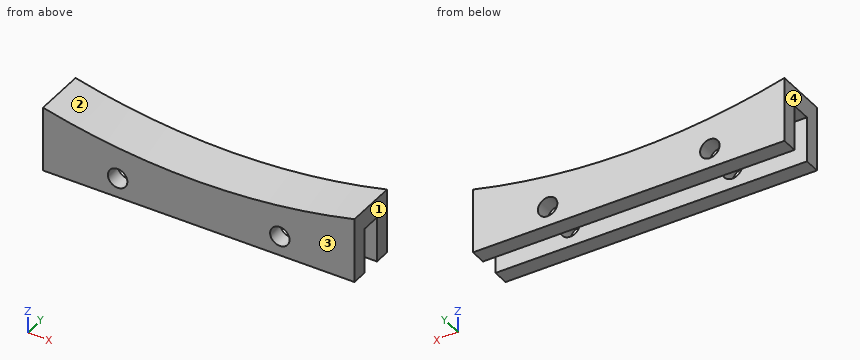
```python
from build123d import *

# Parameters (mm, degrees)
BOSS_EXTRUDE1_DEPTH = 4
SKETCH10_R          = 1.5
SKETCH10_W          = 40
SKETCH10_H          = 6.922711204
CUT_EXTRUDE2_DEPTH  = 31.436460939
SKETCH11_W          = 48
SKETCH11_H          = 1.077288796
BOSS_EXTRUDE2_DEPTH = 8
SKETCH12_W          = 7
SKETCH12_H          = 3.075
CUT_EXTRUDE3_DEPTH  = 52.052699777


with BuildPart() as part:
    # Sketch1 → Boss-Extrude1 (new, symmetric)
    with BuildSketch(Plane(origin=(0, 0, 0), x_dir=(1, 0, 0), z_dir=(0, 1, 0))):
        with BuildLine():
            Line((-20, 0), (0, 0))
            Line((0, 0), (20, 0))
            Line((20, 0), (20, -8))
            Line((20, -8), (24, -8))
            Line((24, -8), (24, -16.922711204))
            ThreePointArc((24, -16.922711204), (0, -14), (-24, -16.922711204))
            Line((-24, -16.922711204), (-24, -8))
            Line((-24, -8), (-20, -8))
            Line((-20, -8), (-20, 0))
        make_face()
    extrude(amount=BOSS_EXTRUDE1_DEPTH, both=True)

    # Sketch10 → Cut-Extrude2 (cut, through all)
    with BuildSketch(Plane(origin=(0, 4, 0), x_dir=(1, 0, 0), z_dir=(0, 1, 0))):
        with Locations(Location((-12.5, -9.922711204, 0), (0, 0, 270))):
            Circle(SKETCH10_R)
        with Locations(Location((12.5, -9.922711204, 0), (0, 0, 270))):
            Circle(SKETCH10_R)
        with Locations((0, -3.461355602)):
            Rectangle(SKETCH10_W, SKETCH10_H)
    extrude(amount=-CUT_EXTRUDE2_DEPTH, mode=Mode.SUBTRACT)

    # Sketch11 → Boss-Extrude2 (add)
    with BuildSketch(Plane(origin=(0, 4, 0), x_dir=(1, 0, 0), z_dir=(0, 1, 0))):
        with Locations((0, -7.461355602)):
            Rectangle(SKETCH11_W, SKETCH11_H)
    extrude(amount=-BOSS_EXTRUDE2_DEPTH)

    # Sketch12 → Cut-Extrude3 (cut, through all)
    with BuildSketch(Plane.ZY.offset(24)):
        with Locations((10.422711204, 0)):
            Rectangle(SKETCH12_W, SKETCH12_H)
    extrude(amount=-CUT_EXTRUDE3_DEPTH, mode=Mode.SUBTRACT)


solid = part.part
```
Design review of the part built by this model. Coordinates are the model's own, in mm. Face numbers are marked on the shaded views. Give positions to 0.01 mm unless a question says otherwise; leave off trailing zeros. Write each loop counter-clockwise with the first axis right and the second up, starting at its lowest first coordinate (ties: lowest second). Pieces come first, ordered by that corner, then holes. Notation, with made-up numbers: (84, 74.5) -> (97, 74.5) arc R6 cw to (97, 85.5) -> close; hole circle Ø7 at (-3, -17.75). An arc over 180 degrees is marked (long way). Answer in a Markdown table with one row per item.
(1) Consider section C-C (x = -12.5). State the section outline as (y, z) points.
Results:
| item | result |
|---|---|
| outline | (-4, 6.92) -> (-1.54, 6.92) -> (-1.54, 8.42) -> (-4, 8.42) -> close; (-4, 11.42) -> (-1.54, 11.42) -> (-1.54, 13.92) -> (1.54, 13.92) -> (1.54, 11.42) -> (4, 11.42) -> (4, 14.78) -> (-4, 14.78) -> close; (1.54, 6.92) -> (4, 6.92) -> (4, 8.42) -> (1.54, 8.42) -> close |
(2) Clearance check with flat-ended pins moving along their axes: pin 1 (5 mm diameter, centred on x = 12.5, z = 9.92, fed in from +Y); pin 2 (1.8 mm diameter, centred on x = 12.5, z = 9.92, fed in from -Y); pin 3 (4 mm diameter, centred on x = 15, y = -2.5, fed in from +Z); pin 4 (3 mm diameter, centred on x = 10.5, y = -3, fed in from +Z). State where each tip first meets the part, or that it passes through.
Results:
| item | result |
|---|---|
| pin 1 | y = 4 |
| pin 2 | through |
| pin 3 | z = 15.46 |
| pin 4 | z = 14.72 |
(3) Consider section D-D (z = 9). State the section outline as (x, y) points, then the cut area to 3 significant figures.
Results:
| item | result |
|---|---|
| outline | (-24, -4) -> (-13.68, -4) -> (-13.68, -1.54) -> (-24, -1.54) -> close; (-24, 1.54) -> (-13.68, 1.54) -> (-13.68, 4) -> (-24, 4) -> close; (-11.32, -4) -> (11.32, -4) -> (11.32, -1.54) -> (-11.32, -1.54) -> close; (-11.32, 1.54) -> (11.32, 1.54) -> (11.32, 4) -> (-11.32, 4) -> close; (13.68, -4) -> (24, -4) -> (24, -1.54) -> (13.68, -1.54) -> close; (13.68, 1.54) -> (24, 1.54) -> (24, 4) -> (13.68, 4) -> close |
| area | 213 mm2 |
(4) To check wall thickness, follow probe 1 along Y at (x, z) = (-2.5, 13.5); probe 2 along X at (y, z) = (2.5, 10.5); probe 3 along X at (y, z) = (3, 8.75). State the ranges of each line that lie inside material, in increasing order.
Results:
| item | result |
|---|---|
| probe 1 | -4 to -1.54, 1.54 to 4 |
| probe 2 | -24 to -13.88, -11.12 to 11.12, 13.88 to 24 |
| probe 3 | -24 to -13.44, -11.56 to 11.56, 13.44 to 24 |
(5) Consider section B-B (y = -2). State the section outline as (x, z) points.
Results:
| item | result |
|---|---|
| outline | (-24, 6.92) -> (24, 6.92) -> (24, 16.92) arc R100 cw to (-24, 16.92) -> close; hole circle Ø3 at (-12.5, 9.92); hole circle Ø3 at (12.5, 9.92) |
(6) Consider section A-A (z = 12.25). State the section outline as (x, y) points.
Results:
| item | result |
|---|---|
| outline | (-24, -4) -> (24, -4) -> (24, -1.54) -> (-24, -1.54) -> close; (-24, 1.54) -> (24, 1.54) -> (24, 4) -> (-24, 4) -> close |
(7) Mouldability with a two-part tool opening along X and no side actions: class the marked faces 1, 2, 3 and 4 as +X half, -X half, draft (parallel to the pull), parting line (faces both ways), or undercut.
Results:
| item | result |
|---|---|
| face 1 | +X half |
| face 2 | undercut |
| face 3 | draft |
| face 4 | -X half |
